Autodesk Inventor part; units mm, degrees
ref_plane "YZ Plane" through (0, 0, 0) normal (1, 0, 0) x (0, 1, 0)
ref_plane "XZ Plane" through (0, 0, 0) normal (0, 1, 0) x (-1, 0, 0)
ref_plane "XY Plane" through (0, 0, 0) normal (0, 0, 1) x (1, 0, 0)
sketch "Sketch1" plane through (0, 0, 0) normal (0, 0, 1) x (1, 0, 0)
  line L0 (-30, 30) -> (30, 30)
  line L1 (30, 30) -> (30, -30)
  line L2 (30, -30) -> (-30, -30)
  line L3 (-30, -30) -> (-30, 30)
  point P0 (0, 0)
  dimension "d0" = 60
  dimension "d1" = 60
  dimension "d2" = 30
  dimension "d3" = 30
extrude "Extrusion1" add sketch "Sketch1" along normal blind 46
sketch "Sketch2" plane through (0, 0, 46) normal (0, 0, 1) x (1, 0, 0)
  circle A0 centre (0, 0) radius 30
  dimension "d14" = 60
extrude "Extrusion2" add sketch "Sketch2" along normal blind 94
fillet "Fillet1" radius 5 1 edges at (-30, 0, 140)
fillet "Fillet2" radius 2 7 edges at (30, 30, 23) (30, -30, 23) (30, 0, 0) (-30, 30, 23) (0, 30, 0) (-30, 0, 0) (0, -30, 0)
sketch "Sketch3" plane through (0, 0, 0) normal (0, 0, -1) x (-1, 0, 0)
  line L0 (30, -30) -> (30, 28)
  line L1 (30, 0) -> (10, 0)
  circle A0 centre (10, 0) radius 4
  point P0 (0, 0)
  dimension "d10" = 20
  dimension "d11" = 8
  dimension "d15" = 0
extrude "Extrusion3" add sketch "Sketch3" along normal blind 30
properties part number "Motor"
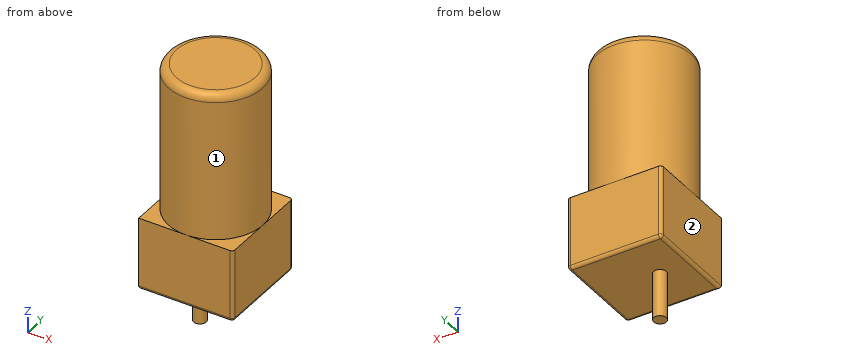
Geometry check sheet. Reference: the model listing, model coordinates, mm. Face numbers are marked on the shaded views. A direction names the side the tool comes from. Coordinates: 2 decimals unless noted, no trailing zeros. Loops run counter-clockwise (first coordinate to the right, second up) from the corner with the lowest first, then second, coordinate; pieces in that order, holes last. Notation, with made-up numbers: (83.5, 79.25) -> (107.5, 79.25) arc R24 cw to (107.5, 103.25) -> close; hole circle Ø5 at (-19.5, -3.5). An arc over 180 degrees is marked (long way). Put each result on its own line as item: value.
1) Cross-section at B-B on z = 81.5. Record the boundary of the cut face in (x, y).
Result set:
outline: circle Ø60 at (0, 0)
2) Gauge pin test, flat ends, axial feed: pin 1 Ø12 at (y, z) = (-2.5, -7.5) entering from +X; pin 2 Ø2 at (x, z) = (-4, 57.5) entering from -Y. Record the tip position at first contact, or that the pin passes through.
Result set:
pin 1: stops at x = -6
pin 2: stops at y = -29.85
3) Cross-section at A-A on z = -16.5. Record the boundary of the cut face in (x, y).
Result set:
outline: circle Ø8 at (-10, 0)
4) Tool access check on the marked faces 1 and 2. Record the directions out of +Z, -Z, +X, -X, +Y, -Y that give a thin tool (end or side, any length) a straight path to the whole face; none if there is none.
Result set:
face 1: +Z
face 2: +Z, -Z, -X, +Y, -Y
5) Thickness scan on line 1 (Y direction, x = 0, z = 118); line 2 (Z direction, x = 2, y = -23); line 3 (Z direction, x = 23, y = 23.5). Record the ranges inside material, lowest first.
Result set:
line 1: y = -30 to 30
line 2: z = 0 to 140
line 3: z = 0 to 46
